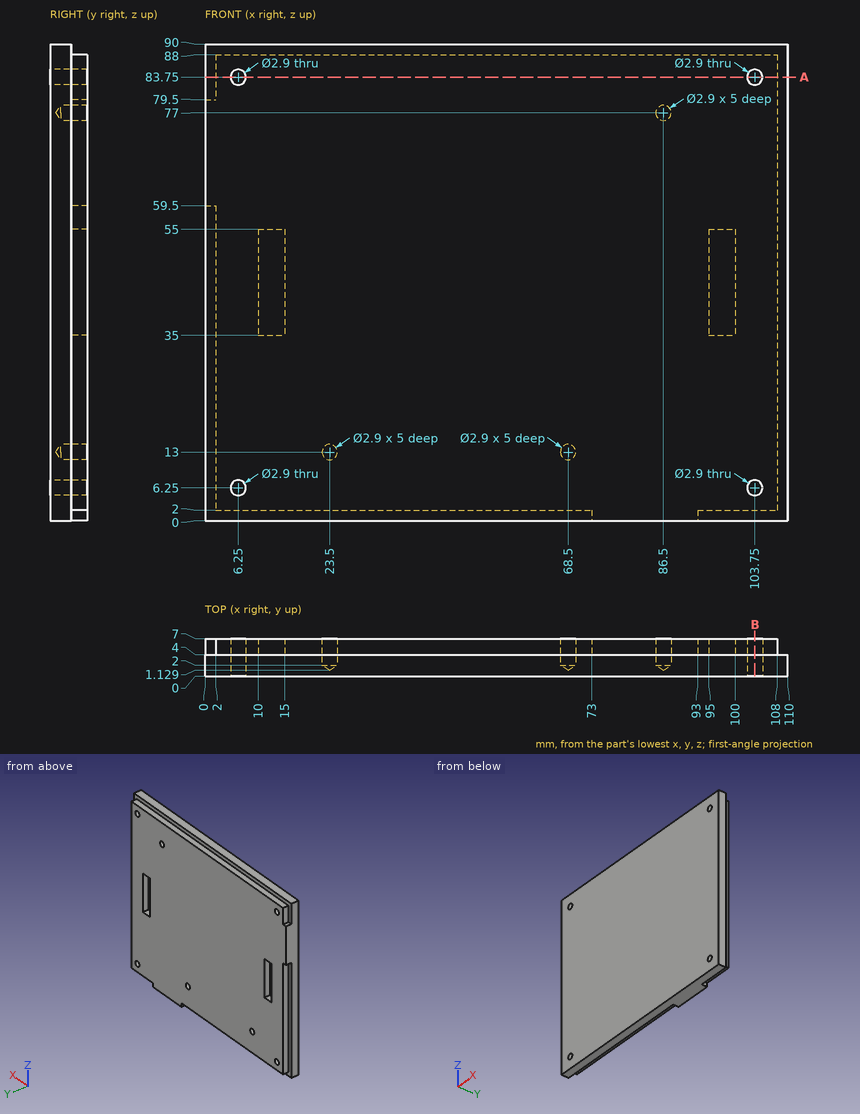
Check sheet for the drawn part. Datum: minimum x, y, z corner. Units: mm. Coordinates: 2 decimals unless noted, no trailing zeros. Order: outer loops, then holes, each group sorted by start corner. A loop starts at its lowest first (then second) coordinate and runs counter-clockwise, first axis right, second up. Notation, with made-up numbers: (-40, 60.5) -> (-27, 60.5) arc R25 cw to (-27, 74.5) -> close; hole circle Ø2 at (-13.5, 71). An arc over 180 degrees is marked (long way). Write each question's results on one line, items separated by ' | '. Start each with the question number.
1) Section check B-B (x = 103.75). Enter the section's corners in (y, z).
2) Section check A-A (z = 83.75). Enter the section's corners in (x, y).
3) Material ranges on line 1 along X through (y, z) = (4.5, 83.75); line 2 along X through (y, z) = (3.1, 13); line 3 along Z through (x, y) = (6.25, 5.25), recorded low to high.
4) Depth check by flat-ended pin: pin 1 (0.9 mm diameter, centred on x = 97, y = 6, fed in from +Z); pin 2 (1.6 mm diameter, centred on x = 0.5, y = 5, fed in from +Z); pin 3 (1.7 mm diameter, centred on x = 23.5, z = 13, fed in from +Y). Enter the tip coordinate at first touch or a pass-through.
Checked values:
1) outline: (0, 0) -> (4, 0) -> (4, 2) -> (7, 2) -> (7, 4.8) -> (0, 4.8) -> close; (0, 7.7) -> (7, 7.7) -> (7, 82.3) -> (0, 82.3) -> close; (0, 85.2) -> (7, 85.2) -> (7, 88) -> (4, 88) -> (4, 90) -> (0, 90) -> close
2) outline: (0, 0) -> (4.8, 0) -> (4.8, 7) -> (2, 7) -> (2, 4) -> (0, 4) -> close; (7.7, 0) -> (102.3, 0) -> (102.3, 7) -> (7.7, 7) -> close; (105.2, 0) -> (110, 0) -> (110, 4) -> (108, 4) -> (108, 7) -> (105.2, 7) -> close
3) line 1: 2 to 4.8, 7.7 to 102.3, 105.2 to 108 | line 2: 0 to 22.05, 24.95 to 67.05, 69.95 to 110 | line 3: 2 to 4.8, 7.7 to 82.3, 85.2 to 88
4) pin 1: z = 88 | pin 2: z = 79.5 | pin 3: y = 1.64
